from build123d import *

# Parameters (mm, degrees)
EXTRUDE_1_DEPTH = 1.5
FILLET_4_R      = 10
FILLET_7_R      = 1.5
FILLET_8_R      = 3
CHAMFER_1_SIZE  = 0.1
FILLET_9_R      = 2
FILLET_10_R     = 0.5


with BuildPart() as part:
    # 草图1 → 凸台-拉伸1 (new, symmetric)
    with BuildSketch(Plane.XY):
        with BuildLine():
            Line((-130, 3.05), (-130, 14.015709241))
            ThreePointArc((-130, 14.015709241), (-134.003306479, 13.533897343), (-138, 13))
            ThreePointArc((-138, 13), (-144, 12), (-150, 13))
            Line((-150, 13), (-156.350852961, 24))
            Line((-156.350852961, 24), (-182, 24))
            Line((-182, 24), (-187.773502692, 14))
            Line((-187.773502692, 14), (-189.773502692, 14))
            Line((-189.773502692, 14), (-192.082903769, 18))
            Line((-192.082903769, 18), (-213.75055535, 18))
            Line((-213.75055535, 18), (-220, 7.175644347))
            Line((-220, 7.175644347), (-220, 5.05))
            Line((-220, 5.05), (-215.5, 5.05))
            Line((-215.5, 5.05), (-215.5, 8.3))
            Line((-215.5, 8.3), (-213, 8.3))
            Line((-213, 8.3), (-210.575128869, 12.5))
            Line((-210.575128869, 12.5), (-195.258330249, 12.5))
            Line((-195.258330249, 12.5), (-192.948929172, 8.5))
            Line((-192.948929172, 8.5), (-186.581793069, 8.5))
            Line((-186.581793069, 8.5), (-184.58993464, 5.05))
            Line((-184.58993464, 5.05), (-174.637306696, 5.05))
            Line((-174.637306696, 5.05), (-177.812733176, 10.55))
            Line((-177.812733176, 10.55), (-181.41450816, 10.55))
            Line((-181.41450816, 10.55), (-182.41450816, 12.282050808))
            Line((-182.41450816, 12.282050808), (-178.824573519, 18.5))
            Line((-178.824573519, 18.5), (-159.526279442, 18.5))
            Line((-159.526279442, 18.5), (-153.637306696, 8.3))
            Line((-153.637306696, 8.3), (-150.937306696, 8.3))
            Line((-150.937306696, 8.3), (-150.937306696, 3.05))
            Line((-150.937306696, 3.05), (-145.837306696, 3.05))
            Line((-145.837306696, 3.05), (-145.837306696, -3.05))
            Line((-145.837306696, -3.05), (-150.937306696, -3.05))
            Line((-150.937306696, -3.05), (-150.937306696, -8.3))
            Line((-150.937306696, -8.3), (-153.637306696, -8.3))
            Line((-153.637306696, -8.3), (-159.526279442, -18.5))
            Line((-159.526279442, -18.5), (-178.824573519, -18.5))
            Line((-178.824573519, -18.5), (-182.41450816, -12.282050808))
            Line((-182.41450816, -12.282050808), (-181.41450816, -10.55))
            Line((-181.41450816, -10.55), (-177.812733176, -10.55))
            Line((-177.812733176, -10.55), (-174.637306696, -5.05))
            Line((-174.637306696, -5.05), (-184.58993464, -5.05))
            Line((-184.58993464, -5.05), (-186.581793069, -8.5))
            Line((-186.581793069, -8.5), (-192.948929172, -8.5))
            Line((-192.948929172, -8.5), (-195.258330249, -12.5))
            Line((-195.258330249, -12.5), (-210.575128869, -12.5))
            Line((-210.575128869, -12.5), (-213, -8.3))
            Line((-213, -8.3), (-215.5, -8.3))
            Line((-215.5, -8.3), (-215.5, -5.05))
            Line((-215.5, -5.05), (-220, -5.05))
            Line((-220, -5.05), (-220, -7.175644347))
            Line((-220, -7.175644347), (-213.75055535, -18))
            Line((-213.75055535, -18), (-192.082903769, -18))
            Line((-192.082903769, -18), (-189.773502692, -14))
            Line((-189.773502692, -14), (-187.773502692, -14))
            Line((-187.773502692, -14), (-182, -24))
            Line((-182, -24), (-156.350852961, -24))
            Line((-156.350852961, -24), (-150, -13))
            ThreePointArc((-150, -13), (-144, -12), (-138, -13))
            ThreePointArc((-138, -13), (-134.003306479, -13.533897343), (-130, -14.015709241))
            Line((-130, -14.015709241), (-130, -3.05))
            Line((-130, -3.05), (-140.837306696, -3.05))
            Line((-140.837306696, -3.05), (-140.837306696, 3.05))
            Line((-140.837306696, 3.05), (-130, 3.05))
        make_face()
    extrude(amount=EXTRUDE_1_DEPTH, both=True)

    # 圆角4
    fillet_4_edges = [part.edges().sort_by_distance(p)[0] for p in [
        (-138, 13, 0),
        (-138, -13, 0),
        (-150, -13, 0),
        (-150, 13, 0),
    ]]
    fillet(fillet_4_edges, radius=FILLET_4_R)

    # 圆角7
    fillet_7_edges = [part.edges().sort_by_distance(p)[0] for p in [
        (-187.773502692, -14, 0),
        (-189.773502692, -14, 0),
        (-210.575128869, -12.5, 0),
        (-195.258330249, -12.5, 0),
        (-186.581793069, -8.5, 0),
        (-181.41450816, -10.55, 0),
        (-182.41450816, -12.282050808, 0),
        (-178.824573519, -18.5, 0),
        (-159.526279442, -18.5, 0),
        (-159.526279442, 18.5, 0),
        (-178.824573519, 18.5, 0),
        (-182.41450816, 12.282050808, 0),
        (-181.41450816, 10.55, 0),
        (-186.581793069, 8.5, 0),
        (-195.258330249, 12.5, 0),
        (-210.575128869, 12.5, 0),
        (-189.773502692, 14, 0),
        (-187.773502692, 14, 0),
    ]]
    fillet(fillet_7_edges, radius=FILLET_7_R)

    # 圆角8
    fillet_8_edges = [part.edges().sort_by_distance(p)[0] for p in [
        (-156.350852961, -24, 0),
        (-182, -24, 0),
        (-192.082903769, -18, 0),
        (-213.75055535, -18, 0),
        (-192.948929172, -8.5, 0),
        (-184.58993464, -5.05, 0),
        (-177.812733176, -10.55, 0),
        (-177.812733176, 10.55, 0),
        (-184.58993464, 5.05, 0),
        (-192.948929172, 8.5, 0),
        (-213.75055535, 18, 0),
        (-192.082903769, 18, 0),
        (-182, 24, 0),
        (-156.350852961, 24, 0),
    ]]
    fillet(fillet_8_edges, radius=FILLET_8_R)

    # 倒角1
    chamfer_1_edges = [part.edges().sort_by_distance(p)[0] for p in [
        (-130, 3.05, 0),
        (-140.837306696, 3.05, 0),
        (-140.837306696, -3.05, 0),
        (-130, -3.05, 0),
        (-220, -5.05, 0),
        (-215.5, -5.05, 0),
        (-150.937306696, -3.05, 0),
        (-145.837306696, -3.05, 0),
        (-145.837306696, 3.05, 0),
        (-150.937306696, 3.05, 0),
        (-215.5, 5.05, 0),
        (-220, 5.05, 0),
    ]]
    chamfer(chamfer_1_edges, length=CHAMFER_1_SIZE)

    # 圆角9
    fillet_9_edges = [part.edges().sort_by_distance(p)[0] for p in [
        (-130, 14.015709241, 0),
        (-130, -14.015709241, 0),
    ]]
    fillet(fillet_9_edges, radius=FILLET_9_R)

    # 圆角10
    fillet_10_edges = [part.edges().sort_by_distance(p)[0] for p in [
        (-174.637306696, -5.05, 0),
        (-174.637306696, 5.05, 0),
    ]]
    fillet(fillet_10_edges, radius=FILLET_10_R)


solid = part.part
Verification items for the finished model (mm, model axes). A direction names the side the tool comes from. Round coordinates to 2 decimals unless told otherwise and drop trailing zeros. Write each loop counter-clockwise with the first axis right and the second up, starting at its lowest first coordinate (ties: lowest second). Pieces come first, ordered by that corner, then holes.
(1) Depth check by flat-ended pin: pin 1 Ø1 at (x, z) = (-144, -1) entering from +Y; pin 2 Ø0.9 at (x, z) = (-148.5, 0) entering from +Y; pin 3 Ø0.9 at (y, z) = (4.5, 0) entering from -X. Enter the tip coordinate at first touch or a pass-through.
Returned:
pin 1: stops at y = 12.04
pin 2: stops at y = 13.53
pin 3: stops at x = -150.94
(2) Mould release check, pull along X, two halves, no side actions. Record for faces 4 (the flat face through (-135, -3.05, 0)), 5 (the flat face through (-169, 18.5, 0)), 6 (the flat face through (-180.639, 15.358, 0.021)), 7 (the flat face through (-145.837, 0, 0)): pulls with the +X half, pulls with the -X half, needs draft (parallel to the pull), parting line crosses it, or undercut.
Returned:
face 4: needs draft
face 5: undercut
face 6: undercut
face 7: pulls with the -X half
(3) Access from +Z, -Z, +X, -X, +Y, -Y to the whole of each face (thin tool, end or side, straight path). Record for faces 1 (the cylindrical face through (-148.542, 13.284, 0.021)), 2 (the flat face through (-214, 8.3, 0)), 3 (the flat face through (-203, -18, 0)).
Returned:
face 1: +Z, -Z, +Y
face 2: +Z, -Z
face 3: +Z, -Z, -X, -Y
(4) Section check C-C (y = 21.5). Enter the section's corners in (x, z).
Returned:
outline: (-183.44, -1.5) - (-154.91, -1.5) - (-154.91, 1.5) - (-183.44, 1.5) - close
(5) Section check A-A (x = -172). Enter the section's corners in (y, z), plus the area to 3 significant figures.
Returned:
outline: (-24, -1.5) - (-18.5, -1.5) - (-18.5, 1.5) - (-24, 1.5) - close; (18.5, -1.5) - (24, -1.5) - (24, 1.5) - (18.5, 1.5) - close
area: 33.0 mm2
(6) Material ranges on line 1 (Y direction, x = -206.5, z = -0.55); line 2 (Y direction, x = -161.5, z = -0.05); line 3 (Y direction, x = -177, z = -0.35), recorded low to high.
Returned:
line 1: y = -18 to -12.5, 12.5 to 18
line 2: y = -24 to -18.5, 18.5 to 24
line 3: y = -24 to -18.5, -9.14 to -5.05, 5.05 to 9.14, 18.5 to 24
(7) Section check B-B (y = 4). Enter the section's corners in (x, z).
Returned:
outline: (-150.94, -1.5) - (-130, -1.5) - (-130, 1.5) - (-150.94, 1.5) - close
